For this review, take the finished solid that the model builds, in its own axes (mm). A direction names the side the tool comes from. Round coordinates to 2 decimals unless told otherwise and drop trailing zeros. Loops run counter-clockwise (first coordinate to the right, second up) from the corner with the lowest first, then second, coordinate; pieces in that order, holes last.
1. Consider section A-A on y = 10. State the section outline as (x, z) points, then the cut area to 3 significant figures.
2. Consider section C-C on x = 25. State the section outline as (y, z) points, then the cut area to 3 significant figures.
3. Consider section B-B on x = 68.7. State the section outline as (y, z) points, then the cut area to 3 significant figures.
4. To check wall thickness, follow line 1 along Y through (x, z) = (3.9, 1.35); line 2 along Y through (x, z) = (68.7, 1.65); line 3 along X through (y, z) = (68, 0.75). State the ranges of each line that lie inside material, in increasing order.
5. Draft analysis for pull direction X (two halves, no side actions). For faces 1 (the flat face through (19, 0, 1)), 2 (the flat face through (76.4, 60, 1)), 3 (the cylindrical face through (0.6, 0.57, 1.48)), state which applies: released by +X, released by -X, zero draft, split by the parting line, or undercut.
6. Consider section D-D on y = 68. State the section outline as (x, z) points, then the cut area to 3 significant figures.
7. Tool access review of faces 4 (the cylindrical face through (0.57, 77.4, 1.48)), 5 (the flat face through (76.4, 30, 1)), 6 (the cylindrical face through (37.47, 14.4, 1.48)): name each direction out of +Z, -Z, +X, -X, +Y, -Y from which nothing blocks a thin tool from reaching the whole face with its end or side.
Autodesk Fusion 360 part; units mm, degrees
sketch "Esquisse1" plane through (0, 0, 0) normal (0, 0, 1) x (1, 0, 0)
  line L0 (88.4, 2) -> (88.4, 76)
  line L1 (86.4, 78) -> (2, 78)
  line L2 (0, 76) -> (0, 2)
  circle A0 centre (3.9, 4) radius 1.75
  circle A1 centre (3.9, 74) radius 1.75
  circle A2 centre (84.5, 74) radius 1.75
  circle A3 centre (84.5, 4) radius 1.75
  arc A4 (0, 2) -> (2, 0) centre (2, 2) ccw
  arc A5 (2, 78) -> (0, 76) centre (2, 76) ccw
  arc A6 (88.4, 76) -> (86.4, 78) centre (86.4, 76) ccw
  arc A7 (86.4, 0) -> (88.4, 2) centre (86.4, 2) ccw
  circle A8 centre (19.7, 10) radius 1.05
  circle A9 centre (68.7, 10) radius 1.05
  circle A10 centre (19.7, 68) radius 1.05
  circle A11 centre (68.7, 68) radius 1.05
  line L3 (51.9, 2) -> (51.9, 13)
  line L4 (49.9, 15) -> (38.9, 15)
  line L5 (36.9, 13) -> (36.9, 2)
  line L6 (34.9, 0) -> (2, 0)
  line L7 (86.4, 0) -> (53.9, 0)
  arc A12 (34.9, 0) -> (36.9, 2) centre (34.9, 2) ccw
  arc A13 (51.9, 2) -> (53.9, 0) centre (53.9, 2) ccw
  arc A14 (51.9, 13) -> (49.9, 15) centre (49.9, 13) ccw
  arc A15 (38.9, 15) -> (36.9, 13) centre (38.9, 13) ccw
  circle A16 centre (58.4, 28) radius 1.05
  circle A17 centre (25, 68) radius 1.3
  circle A18 centre (25, 14) radius 1.3
  line L8 (57.9, 28) -> (56.9, 28)
  line L9 (56.4, 28.5) -> (56.4, 31.5)
  line L10 (56.9, 32) -> (57.9, 32)
  line L11 (58.4, 31.5) -> (58.4, 28.5)
  arc A19 (56.4, 28.5) -> (56.9, 28) centre (56.9, 28.5) ccw
  arc A20 (56.9, 32) -> (56.4, 31.5) centre (56.9, 31.5) ccw
  arc A21 (58.4, 31.5) -> (57.9, 32) centre (57.9, 31.5) ccw
  arc A22 (57.9, 28) -> (58.4, 28.5) centre (57.9, 28.5) ccw
  line L12 (77.9, 28) -> (76.9, 28)
  arc A23 (77.9, 28) -> (78.4, 28.5) centre (77.9, 28.5) ccw
  line L13 (78.4, 31.5) -> (78.4, 28.5)
  line L14 (76.4, 28.5) -> (76.4, 31.5)
  arc A24 (76.4, 28.5) -> (76.9, 28) centre (76.9, 28.5) ccw
  line L15 (76.9, 32) -> (77.9, 32)
  arc A25 (78.4, 31.5) -> (77.9, 32) centre (77.9, 31.5) ccw
  arc A26 (76.9, 32) -> (76.4, 31.5) centre (76.9, 31.5) ccw
  line L16 (57.9, 58) -> (56.9, 58)
  arc A27 (57.9, 58) -> (58.4, 58.5) centre (57.9, 58.5) ccw
  line L17 (58.4, 61.5) -> (58.4, 58.5)
  line L18 (56.4, 58.5) -> (56.4, 61.5)
  arc A28 (56.4, 58.5) -> (56.9, 58) centre (56.9, 58.5) ccw
  line L19 (56.9, 62) -> (57.9, 62)
  arc A29 (58.4, 61.5) -> (57.9, 62) centre (57.9, 61.5) ccw
  arc A30 (56.9, 62) -> (56.4, 61.5) centre (56.9, 61.5) ccw
  line L20 (77.9, 58) -> (76.9, 58)
  arc A31 (77.9, 58) -> (78.4, 58.5) centre (77.9, 58.5) ccw
  line L21 (78.4, 61.5) -> (78.4, 58.5)
  line L22 (76.4, 58.5) -> (76.4, 61.5)
  arc A32 (76.4, 58.5) -> (76.9, 58) centre (76.9, 58.5) ccw
  line L23 (76.9, 62) -> (77.9, 62)
  arc A33 (78.4, 61.5) -> (77.9, 62) centre (77.9, 61.5) ccw
  arc A34 (76.9, 62) -> (76.4, 61.5) centre (76.9, 61.5) ccw
  point P0 (88.4, 0)
  point P1 (0, 78)
  point P2 (36.9, 0)
  point P3 (36.9, 15)
  point P4 (58.4, 28)
  point P5 (56.4, 28)
  point P6 (58.4, 32)
  dimension "d1" = 78
  dimension "d2" = 88.4
  dimension "d3" = 3.5
  dimension "d4" = 3.9
  dimension "d6" = 3.5
  dimension "d8" = 4
  dimension "d9" = 3.5
  dimension "d10" = 4
  dimension "d11" = 3.9
  dimension "d12" = 3.5
  dimension "d13" = 3.9
  dimension "d15" = 2
  dimension "d16" = 2
  dimension "d17" = 2
  dimension "d18" = 2
  dimension "d21" = 2.1
  dimension "d24" = 49
  dimension "d25" = 58
  dimension "d28" = 19.7
  dimension "d30" = 15
  dimension "d31" = 36.9
  dimension "d33" = 2
  dimension "d34" = 2
  dimension "d35" = 2
  dimension "d36" = 2
  dimension "d37" = 15
  dimension "d41" = 2.1
  dimension "d44" = 20
  dimension "d45" = 30
  dimension "d46" = 30
  dimension "d47" = 50
  dimension "d48" = 2.6
  dimension "d51" = 0
  dimension "d52" = -54
  dimension "d53" = 10
  dimension "d54" = 25
  dimension "d55" = 2
  dimension "d56" = 4
  dimension "d57" = 0.5
extrude "Extrusion1" add sketch "Esquisse1" along normal blind 3 contours L0 L1 L2 A4 A5 A6 A7 L3 L4 L5 L6 L7 A12 A13 A14 A15 | A16 L8 L11 A22 picked at (58.8173, 27.529)
Resolved:
1. outline: (0, 0) - (18.65, 0) - (18.65, 3) - (0, 3) - close; (20.75, 0) - (36.9, 0) - (36.9, 3) - (20.75, 3) - close; (51.9, 0) - (67.65, 0) - (67.65, 3) - (51.9, 3) - close; (69.75, 0) - (88.4, 0) - (88.4, 3) - (69.75, 3) - close
1. area: 208 mm2
2. outline: (0, 0) - (12.7, 0) - (12.7, 3) - (0, 3) - close; (15.3, 0) - (66.7, 0) - (66.7, 3) - (15.3, 3) - close; (69.3, 0) - (78, 0) - (78, 3) - (69.3, 3) - close
2. area: 218 mm2
3. outline: (0, 0) - (8.95, 0) - (8.95, 3) - (0, 3) - close; (11.05, 0) - (66.95, 0) - (66.95, 3) - (11.05, 3) - close; (69.05, 0) - (78, 0) - (78, 3) - (69.05, 3) - close
3. area: 221 mm2
4. line 1: y = 0 to 2.25, 5.75 to 72.25, 75.75 to 78
4. line 2: y = 0 to 8.95, 11.05 to 66.95, 69.05 to 78
4. line 3: x = 0 to 18.65, 20.75 to 23.7, 26.3 to 67.65, 69.75 to 88.4
5. face 1: zero draft
5. face 2: undercut
5. face 3: released by -X
6. outline: (0, 0) - (18.65, 0) - (18.65, 3) - (0, 3) - close; (20.75, 0) - (23.7, 0) - (23.7, 3) - (20.75, 3) - close; (26.3, 0) - (67.65, 0) - (67.65, 3) - (26.3, 3) - close; (69.75, 0) - (88.4, 0) - (88.4, 3) - (69.75, 3) - close
6. area: 245 mm2
7. face 4: +Z, -Z, -X, +Y
7. face 5: +Z, -Z
7. face 6: +Z, -Z, -Y
